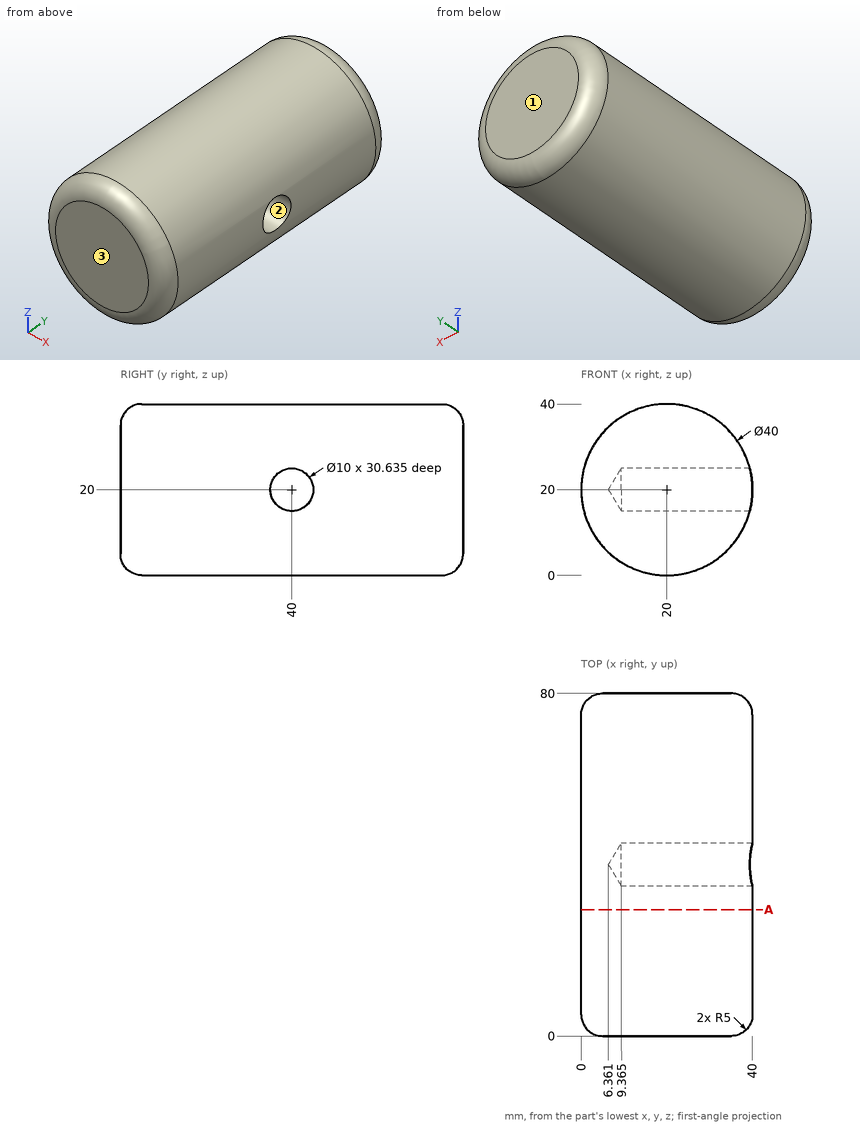
Verification items for this drawing (mm, ordinates from the low corner). Give positions to 0.01 mm unless a question says otherwise; leave off trailing zeros. Loops run counter-clockwise (first coordinate to the right, second up) from the corner with the lowest first, then second, coordinate; pieces in that order, holes last. Notation, with made-up numbers: (74.25, -9) - (122.25, -9) arc R34 ccw to (122.25, 28) - close; hole circle Ø10 at (51.5, 89.25). An arc over 180 degrees is marked (long way). Write item = value, one per line. Start each with the question number.
Q1. Thickness scan on line 1 (Z direction, x = 26, y = 40); line 2 (Y direction, x = 5, z = 23.5); line 3 (Z direction, x = 30.5, y = 36). Record the ranges inside material, lowest first.
Q2. Cross-section at A-A, the plane y = 29.5. Enter the section's corners in (x, z).
Q3. Depth check by flat-ended pin: P1, Ø12, axis at x = 30, z = 8, coming from the -Y side; P2, Ø10, axis at x = 22, y = 39, coming from the +Z side; P3, Ø8, axis at y = 17.5, z = 12.5, coming from the -X side; P4, Ø3, axis at x = 27, y = 59.5, coming from the +Z side. Enter the tip coordinate at first touch or a pass-through.
Q4. Mould release check, pull along Y, two halves, no side actions. Record for the marked faces 1, 2 and 3: released by +Y, released by -Y, zero draft, split by the parting line, or undercut.
Answer key:
q1.line_1 = 0.92 to 15, 25 to 39.08
q1.line_2 = 0.02 to 79.98
q1.line_3 = 2.98 to 17, 23 to 37.02
q2.outline = circle Ø40 at (20, 20)
q3.P1 = 0
q3.P2 = 40
q3.P3 = 0.31
q3.P4 = 39.23
q4.face_1 = released by +Y
q4.face_2 = undercut
q4.face_3 = released by -Y
